Here's how the part is built. I have some questions about the finished solid (model axes, mm). Face numbers are marked on the shaded views. A direction names the side the tool comes from. Round coordinates to 2 decimals unless told otherwise and drop trailing zeros. Write each loop counter-clockwise with the first axis right and the second up, starting at its lowest first coordinate (ties: lowest second). Pieces come first, ordered by that corner, then holes. Notation, with made-up numbers: (6, 41.5) -> (61, 41.5) arc R6 ccw to (61, 46.5) -> close; hole circle Ø9 at (4, 15.5). An arc over 180 degrees is marked (long way). Put each result on its own line as item: value. Start each with the question number.
1) We'd pull the mould along Z, two halves only. Please class the marked faces 3, 4 and 5: released by +Z, released by -Z, zero draft, split by the parting line, or undercut.
2) If I drill on line 1 along Z through (x, y) = (-62, 5); line 2 along X through (y, z) = (4, 72.5); line 3 along X through (y, z) = (-10, 7), over which ranges is the centre line in solid material (lowest first)? Write a range as [from, to].
3) Will these pins go through, and if not, where does the flat tip stop? P1, Ø10, axis at x = 40.5, y = -9, coming from the +Z side; P2, Ø1.5, axis at y = 8, z = 106, coming from the +X side; P3, Ø1, axis at y = -10.5, z = 46, coming from the +X side.
4) I want a section at C-C, the plane y = 0. List the corners of the cut face in (x, z) for me.
5) I want a section at A-A, the plane y = -11. List the corners of the cut face in (x, z) for me, then the cut area to 3 significant figures.
6) Which directions (+Z, -Z, +X, -X, +Y, -Y) give clear straight access to the entire face, cutting with the end or side of a thin tool? Please do the marked faces 1 and 2.
7) I want a section at B-B, the plane x = 37.5. List the corners of the cut face in (y, z) for me.
from build123d import *

# Parameters (mm, degrees)
F1_R          = 15
F4_DEPTH      = 15.0010001
F4_DEPTH_BACK = 15.0010001


with BuildPart() as f2:
    # F2: sweep along a path in F0
    with BuildLine(Plane.XZ) as f2_path:
        Line((0, -12.9099444874), (-62.8431858703, 3.3160963325))
        ThreePointArc((-62.8431858703, 3.3160963325), (-80.2682122339, 15.6678713866), (-85.0590780928, 36.4824214677))
        Line((-85.0590780928, 36.4824214677), (-79.7831982043, 74.5449074598))
        ThreePointArc((-79.7831982043, 74.5449074598), (-66.4329303758, 99.2165061576), (-40.1620085743, 109.052974075))
        Line((-40.1620085743, 109.052974075), (0, 109.052974075))
    # F1 (on Right) → F2 (sweep)
    with BuildSketch(Plane.YZ):
        with Locations((0, 109.052974075)):
            Circle(F1_R)
    sweep(path=f2_path.line)

    # F3: sweep along a path in F0
    with BuildLine(Plane.XZ) as f3_path:
        Line((0, 109.052974075), (40.1620085743, 109.052974075))
        ThreePointArc((40.1620085743, 109.052974075), (66.4329303758, 99.2165061576), (79.7831982043, 74.5449074598))
        Line((79.7831982043, 74.5449074598), (85.0590780928, 36.4824214677))
        ThreePointArc((85.0590780928, 36.4824214677), (80.2682122339, 15.6678713866), (62.8431858703, 3.3160963325))
        Line((62.8431858703, 3.3160963325), (0, -12.9099444874))
    # F1 (on Right) → F3 (sweep)
    with BuildSketch(Plane.YZ):
        with Locations((0, 109.052974075)):
            Circle(F1_R)
    sweep(path=f3_path.line)

    # F0 (on Front) → F4 (cut, two sides)
    with BuildSketch(Plane.XZ) as f4_sk:
        with BuildLine():
            Line((0, -12.9099444874), (50, 0))
            ThreePointArc((50, 0), (0, 50), (-50, 0))
            Line((-50, 0), (0, -12.9099444874))
        make_face()
        with BuildLine():
            ThreePointArc((-50, 0), (0, -50), (50, 0))
            Line((50, 0), (0, -12.9099444874))
            Line((0, -12.9099444874), (-50, 0))
        make_face()
    extrude(amount=-F4_DEPTH, mode=Mode.SUBTRACT)
    extrude(f4_sk.sketch, amount=F4_DEPTH_BACK, mode=Mode.SUBTRACT)


solid = f2.part
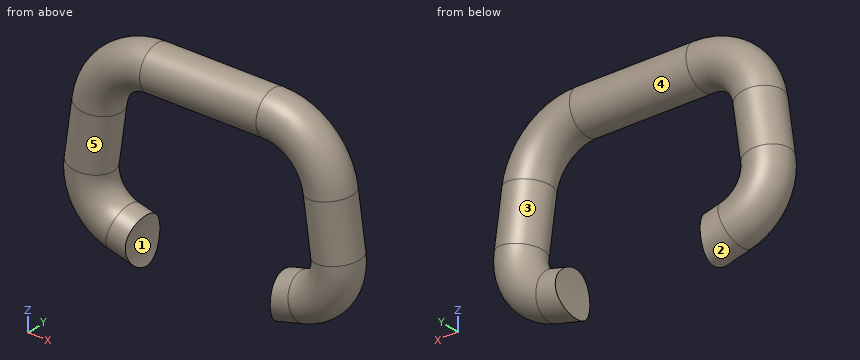
Findings:
1. face 3: undercut
1. face 4: split by the parting line
1. face 5: undercut
2. line 1: z = [-11.51, 17.97], [82.9, 118.6]
2. line 2: x = [-94.66, -65.47], [65.47, 94.66]
2. line 3: x = [-87.79, -49.51], [49.51, 87.79]
3. P1: stops at z = 123.51
3. P2: stops at x = 78.68
3. P3: stops at x = 95.03
4. outline: (-99.92, 38.54) arc R45 ccw to (-66.59, -11.21) -> (-47.31, -16.19) arc R50 cw to (-47.73, 14.9) -> (-59.09, 17.84) arc R15 cw to (-70.2, 34.42) -> (-64.93, 72.49) arc R25 cw to (-40.16, 94.05) -> (40.16, 94.05) arc R25 cw to (64.93, 72.49) -> (70.2, 34.42) arc R15 cw to (59.09, 17.84) -> (47.73, 14.9) arc R50 cw to (47.31, -16.19) -> (66.59, -11.21) arc R45 ccw to (99.92, 38.54) -> (94.64, 76.6) arc R55 ccw to (40.16, 124.05) -> (-40.16, 124.05) arc R55 ccw to (-94.64, 76.6) -> close
5. outline: (-95.16, 37.88) arc R40.2 ccw to (-65.39, -6.56) -> (-48.81, -10.84) arc R50 cw to (-48.94, 10.26) -> (-60.29, 13.19) arc R19.8 cw to (-74.96, 35.08) -> (-69.68, 73.14) arc R29.8 cw to (-40.16, 98.85) -> (40.16, 98.85) arc R29.8 cw to (69.68, 73.14) -> (74.96, 35.08) arc R19.8 cw to (60.29, 13.19) -> (48.94, 10.26) arc R50 cw to (48.81, -10.84) -> (65.39, -6.56) arc R40.2 ccw to (95.16, 37.88) -> (89.88, 75.95) arc R50.2 ccw to (40.16, 119.25) -> (-40.16, 119.25) arc R50.2 ccw to (-89.88, 75.95) -> close
5. area: 7,880 mm2
6. face 1: +Y, -Y
6. face 2: none
7. outline: circle Ø30 at (0, 109.05)
